Verification items for the finished model (mm, model axes). Coordinates: 2 decimals unless noted, no trailing zeros. Order: outer loops, then holes, each group sorted by start corner. A loop starts at its lowest first (then second) coordinate and runs counter-clockwise, first axis right, second up. Notation, with made-up numbers: (-4, 80.5) -> (2, 80.5) arc R10 cw to (2, 90.5) -> close; hole circle Ø4 at (60.5, -5.5). An arc over 180 degrees is marked (long way). Use CSV: the item, a comma, the result in double quotes. Start each with the question number.
1) Scan lines: line 1 along X through (y, z) = (-1.5, 13); line 2 along X through (y, z) = (-0.15, 1); line 3 along Z through (x, y) = (34, -0.35). Record each from-to range of solid material in increasing order.
2) Sectioned sample at A-A on y = -0.45. Record the boundary of the cut face in (x, z).
3) Sectioned sample at B-B on z = 2.5. Record the boundary of the cut face in (x, y).
4) Go/stop test with flat-tipped pins: pin 1 (0.8 mm diameter, centred on x = 37.5, y = -0.5, fed in from -Z); pin 2 (0.5 mm diameter, centred on y = -0.5, z = -13.5, fed in from +X). Record where each tip stops, or that it passes through.
from build123d import *

# Parameters (mm, degrees)
F0_W     = 68
F0_H     = 45
F1_DEPTH = 1.5875
F2_W     = 8.9957
F2_H     = 29
F2_W_2   = 9.0043
F3_DEPTH = 25.4
F4_D     = 3
F5_W     = 1
F5_H     = 16
F6_DEPTH = 25.4


with BuildPart() as f1:
    # F0 (on Front) → F1 (new body)
    with BuildSketch(Plane.XZ):
        with Locations((6.343424, -1.337832)):
            Rectangle(F0_W, F0_H)
    extrude(amount=F1_DEPTH)

    # F2 (on face) → F3 (cut)
    with BuildSketch(Plane.XZ.offset(1.5875)):
        with Locations((-23.158726, -9.337832)):
            Rectangle(F2_W, F2_H)
        with Locations((35.841274, -9.337832)):
            Rectangle(F2_W_2, F2_H)
    extrude(amount=-F3_DEPTH, mode=Mode.SUBTRACT)

    # F4 (through all)
    with Locations(Plane.XZ.offset(1.5875)):
        with Locations((-23.753476, 14.162168), (36.444524, 14.162168)):
            Hole(F4_D / 2)

    # F5 (on face) → F6 (cut)
    with BuildSketch(Plane.XZ.offset(1.5875)):
        with Locations((-27.156576, 13.162168)):
            Rectangle(F5_W, F5_H)
        with Locations((39.843424, 13.162168)):
            Rectangle(F5_W, F5_H)
    extrude(amount=-F6_DEPTH, mode=Mode.SUBTRACT)


solid = f1.part
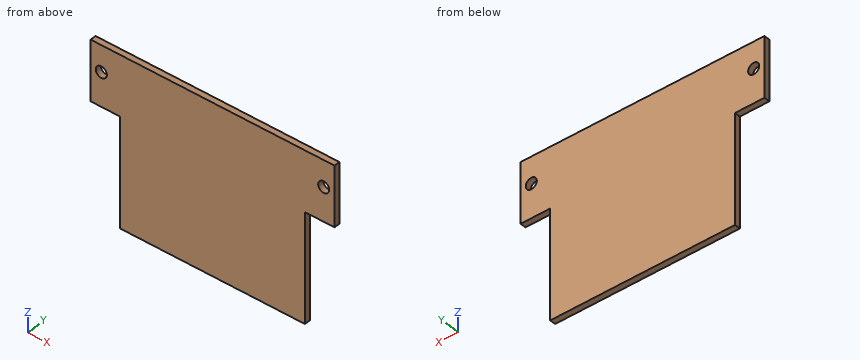
Answers follow:
1,line 1,"x = -26.66 to -24.7, -22.81 to 35.5, 37.39 to 39.34"
1,line 2,"x = -18.66 to 31.34"
1,line 3,"z = 5.16 to 21.16"
2,outline,"(-26.66, 5.16) -> (-18.66, 5.16) -> (-18.66, -23.84) -> (31.34, -23.84) -> (31.34, 5.16) -> (39.34, 5.16) -> (39.34, 21.16) -> (-26.66, 21.16) -> close; hole circle Ø3 at (-23.75, 14.16); hole circle Ø3 at (36.44, 14.16)"
3,outline,"(-18.66, -1.59) -> (31.34, -1.59) -> (31.34, 0) -> (-18.66, 0) -> close"
4,pin 1,"stops at z = 5.16"
4,pin 2,"stops at x = 31.34"
